Geometry check sheet. Reference: the model listing, model coordinates, mm. Face numbers are marked on the shaded views. A direction names the side the tool comes from. Coordinates: 2 decimals unless noted, no trailing zeros. Write each loop counter-clockwise with the first axis right and the second up, starting at its lowest first coordinate (ties: lowest second). Pieces come first, ordered by that corner, then holes. Notation, with made-up numbers: (-1.75, -8) -> (44.25, -8) arc R30 cw to (44.25, 16) -> close; hole circle Ø5 at (38.5, 26.5). An arc over 180 degrees is marked (long way). Answer as CSV lines item,"result".
Autodesk Inventor part; units mm, degrees
ref_plane "YZ Plane" through (0, 0, 0) normal (1, 0, 0) x (0, 1, 0)
ref_plane "XZ Plane" through (0, 0, 0) normal (0, 1, 0) x (-1, 0, 0)
ref_plane "XY Plane" through (0, 0, 0) normal (0, 0, 1) x (1, 0, 0)
sketch "スケッチ1" plane through (0, 0, 0) normal (0, 0, 1) x (1, 0, 0)
  circle A0 centre (0, 0) radius 1.5
  dimension "d0" = 3
extrude "押し出し1" add sketch "スケッチ1" along normal blind 6.25
sketch "スケッチ2" plane through (0, 0, 6.25) normal (0, 0, 1) x (1, 0, 0)
  circle A0 centre (0, 0) radius 1.5
  circle A1 centre (0, 0) radius 3
  dimension "d3" = 6
extrude "押し出し2" add sketch "スケッチ2" along normal blind 1.75 contours A0 | A1
thread "ねじ1"
chamfer "面取り1" distance 1.5 angle 45 1 edges at (-3, 0, 6.25)
properties part number "SB　8mm皿ネジ" material "Steel, Mild"
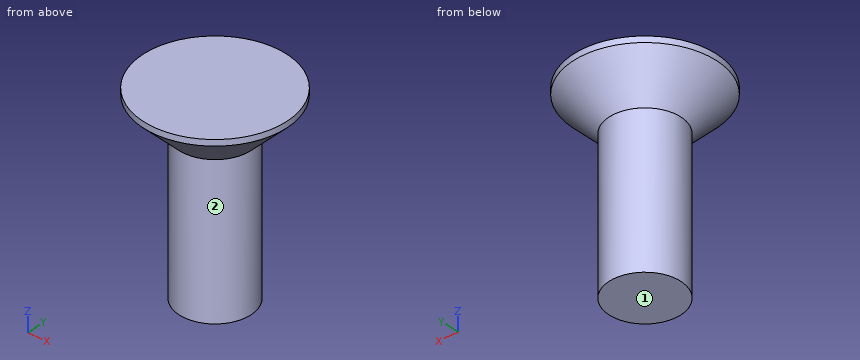
Item 1: Depth check by flat-ended pin: pin 1 Ø2 at (x, z) = (-0.5, 5.5) entering from +Y; pin 2 Ø2 at (y, z) = (-1, 1) entering from +X; pin 3 Ø3 at (y, z) = (0.5, 6) entering from +X. Enter the tip coordinate at first touch or a pass-through.
Responses:
pin 1,"stops at y = 1.7"
pin 2,"stops at x = 1.5"
pin 3,"stops at x = 2.72"
Item 2: Cross-section at C-C, the plane z = 5. Record the cut outline in (x, y), plus the area to 3 significant figures.
Responses:
outline,"circle Ø3 at (0, 0)"
area,"7.07 mm2"
Item 3: Thickness scan on probe 1 along Z at (x, y) = (2, -1.3); probe 2 along Z at (x, y) = (-1.6, -1.8); probe 3 along X at (y, z) = (0.05, 6). Record the ranges inside material, lowest first.
Responses:
probe 1,"z = 7.13 to 8"
probe 2,"z = 7.16 to 8"
probe 3,"x = -1.5 to 1.5"
Item 4: Set-up check for the marked faces 1 and 2: record each of +Z, -Z, +X, -X, +Y, -Y from which the full face is reachable in a straight line by a thin tool's end or side.
Responses:
face 1,"-Z, +X, -X, +Y, -Y"
face 2,"-Z"
Item 5: Cross-section at D-D, the plane z = 7.5. Record the cut outline in (x, y).
Responses:
outline,"circle Ø5.5 at (0, 0)"
